from build123d import *

# Parameters (mm, degrees)
F0_W     = 150.6762728095
F0_H     = 115.9463040531
F1_DEPTH = 25.4
F2_R     = 5
F3_SIZE  = 5
F4_T     = 2.5


# Not quite as in the source:
# - a shell that OpenCascade refuses in one call is made with other operations: the cavity is built on its own and cut out


with BuildPart() as f1:
    # F0 (on Top) → F1 (new body)
    with BuildSketch(Plane.XY):
        with Locations((-0.7436312735, 18.0544536561)):
            Rectangle(F0_W, F0_H)
    extrude(amount=F1_DEPTH)

    # F2
    f2_edges = [f1.edges().sort_by_distance(p)[0] for p in [
        (-76.081768, -39.918698, 12.7),
        (74.594505, -39.918698, 12.7),
        (74.594505, 76.027606, 12.7),
    ]]
    fillet(f2_edges, radius=F2_R)

    # F3
    f3_edges = [f1.edges().sort_by_distance(p)[0] for p in [
        (-76.081768, 20.554454, 25.4),
        (-74.617302, -38.454232, 25.4),
        (-3.243631, 76.027606, 25.4),
        (-0.743631, -39.918698, 25.4),
        (73.130039, 74.56314, 25.4),
        (73.130039, -38.454232, 25.4),
        (74.594505, 18.054454, 25.4),
    ]]
    chamfer(f3_edges, length=F3_SIZE)

    # F4: shell of thickness 2.5, made by hand


with BuildPart() as f4_core1:
    # F4_t2: copy of F1
    add(f1.part)

    # the walls: a layer under each face that stays
    f4_faces = [f4_core1.faces().sort_by_distance(p)[0] for p in [
        (-76.0817676783, 20.5544536561, 10.2),
        (-74.6173015842, -38.4542322764, 10.2),
        (-73.5817676783, 20.5544536561, 22.9),
        (-3.2436312735, 76.0276056826, 10.2),
        (-72.8495346312, -36.6864653234, 22.9),
        (-0.7436312735, -39.9186983705, 10.2),
        (-3.2436312735, 73.5276056826, 22.9),
        (-0.7436312735, 18.0544536561, 25.4),
        (73.1300390372, 74.5631395885, 10.2),
        (73.1300390372, -38.4542322764, 10.2),
        (74.5945051312, 18.0544536561, 10.2),
        (-0.7436312735, -37.4186983705, 22.9),
        (71.3622720842, 72.7953726356, 22.9),
        (72.0945051312, 18.0544536561, 22.9),
        (71.3622720842, -36.6864653234, 22.9),
    ]]
    thicken(f4_faces, amount=-F4_T, mode=Mode.SUBTRACT)


with BuildPart() as f1_1:
    add(f1.part)

    # what is left inside the walls is the cavity
    f4_cavity = [f4_core1.part.solids().sort_by_distance(p)[0] for p in [
        (-0.743631, -0.436597, 0.025),
    ]]
    add(f4_cavity, mode=Mode.SUBTRACT)


solid = f1_1.part
Geometry check sheet. Reference: the model listing, model coordinates, mm. A direction names the side the tool comes from. Coordinates: 2 decimals unless noted, no trailing zeros. Order: outer loops, then holes, each group sorted by start corner. A loop starts at its lowest first (then second) coordinate and runs counter-clockwise, first axis right, second up. Notation, with made-up numbers: (-15.75, 26) -> (24.25, 26) arc R14 ccw to (24.25, 46) -> close; hole circle Ø9 at (59.5, 14). An arc over 180 degrees is marked (long way). Use a Markdown table: item, result. Add a question column.
1. Cross-section at A-A (z = 10). Enter the section's corners in (x, y).
2. Mould release check, pull along X, two halves, no side actions. Record for faces 3 (the face through (-73.547, 19.778, 22.935)), 4 (the face through (-3, 73.528, 10)), 5 (the face through (-2, -39.919, 10)), 6 (the face through (71.357, -36.642, 22.935)): pulls with the +X half, pulls with the -X half, needs draft (parallel to the pull), parting line crosses it, or undercut.
3. Set-up check for faces 1 (the face through (-2.996, 71.735, 21.157)), 2 (the face through (-72.806, -36.681, 22.935)): record each of +Z, -Z, +X, -X, +Y, -Y from which the full face is reachable in a straight line by a thin tool's end or side.
4. Cross-section at B-B (y = 31.5). Enter the section's corners in (x, z), and give its area (3 significant figures).
5. Go/stop test with a flat-tipped pin: pin 1 Ø5 at (x, y) = (30, 24.5) entering from -Z. Record where the tip stops, or that it passes through.
6. Cross-section at C-C (x = -58). Enter the section's corners in (y, z).
7. Material ranges on L1, parallel to Y at x = 13, z = 11.75; L2, parallel to X at y = -28.5, z = 3.5; L3, parallel to Z at x = 62.5, y = 23, recorded low to high.
Filled sheet:
| question | item | result |
|---|---|---|
| 1 | outline | (-76.08, -34.92) arc R5 ccw to (-71.08, -39.92) -> (69.59, -39.92) arc R5 ccw to (74.59, -34.92) -> (74.59, 71.03) arc R5 ccw to (69.59, 76.03) -> (-76.08, 76.03) -> close; hole (-73.58, -34.92) arc R2.5 ccw to (-71.08, -37.42) -> (69.59, -37.42) arc R2.5 ccw to (72.09, -34.92) -> (72.09, 71.03) arc R2.5 ccw to (69.59, 73.53) -> (-73.58, 73.53) -> close |
| 2 | face 3 | pulls with the -X half |
| 2 | face 4 | undercut |
| 2 | face 5 | needs draft |
| 2 | face 6 | pulls with the +X half |
| 3 | face 1 | -Z |
| 3 | face 2 | +Z, -X, -Y |
| 4 | outline | (-76.08, 0) -> (-73.58, 0) -> (-73.58, 19.36) -> (-70.05, 22.9) -> (68.56, 22.9) -> (72.09, 19.36) -> (72.09, 0) -> (74.59, 0) -> (74.59, 20.4) -> (69.59, 25.4) -> (-71.08, 25.4) -> (-76.08, 20.4) -> close |
| 4 | area | 479 mm2 |
| 5 | pin 1 | z = 22.9 |
| 6 | outline | (-39.92, 0) -> (-37.42, 0) -> (-37.42, 19.36) -> (-33.88, 22.9) -> (69.99, 22.9) -> (73.53, 19.36) -> (73.53, 0) -> (76.03, 0) -> (76.03, 20.4) -> (71.03, 25.4) -> (-34.92, 25.4) -> (-39.92, 20.4) -> close |
| 7 | L1 | -39.92 to -37.42, 73.53 to 76.03 |
| 7 | L2 | -76.08 to -73.58, 72.09 to 74.59 |
| 7 | L3 | 22.9 to 25.4 |
